Autodesk Inventor part; units mm, degrees
ref_plane "YZ Plane" through (0, 0, 0) normal (1, 0, 0) x (0, 1, 0)
ref_plane "XZ Plane" through (0, 0, 0) normal (0, 1, 0) x (-1, 0, 0)
ref_plane "XY Plane" through (0, 0, 0) normal (0, 0, 1) x (1, 0, 0)
sketch "Sketch1" plane through (0, 0, 0) normal (0, 0, 1) x (1, 0, 0)
  circle A0 centre (0, 0) radius 5
  dimension "d0" = 10
extrude "Extrusion1" add sketch "Sketch1" along normal blind 1
sketch "Sketch2" plane through (0, 0, 1) normal (0, 0, 1) x (1, 0, 0)
  circle A0 centre (0, 0) radius 1.5
  circle A1 centre (0, 0) radius 2
  dimension "d3" = 3
  dimension "d4" = 4
extrude "Extrusion2" cut sketch "Sketch2" against normal blind 1.5 contours A0
extrude "Extrusion3" add sketch "Sketch2" along normal blind 2
mirror "Mirror2" about plane through (0, 0, 0) normal (0, 0, -1)
properties part number "einzel_element"
Source: CAD feature listing. Evaluate the final solid. Frame: model axes, mm. A direction names the side the tool comes from. Round coordinates to 2 decimals unless told otherwise and drop trailing zeros. Loops run counter-clockwise (first coordinate to the right, second up) from the corner with the lowest first, then second, coordinate; pieces in that order, holes last. Notation, with made-up numbers: (52.5, -18.75) - (104.5, -18.75) arc R28 ccw to (104.5, 8.25) - close; hole circle Ø7 at (35.25, 37.25). An arc over 180 degrees is marked (long way). Write item = value, one per line. Start each with the question number.
(1) Set-up query: faces 4 (the face through (0, 2, 2)), 5 (the face through (-1.08, -4.88, 0.01)). Return all of +Z, -Z, +X, -X, +Y, -Y with unobstructed straight access to the full face (end or side cutting, diameter ignored); none if empty.
(2) Section query C-C, the plane z = 1.85. Output: boundary loops of the cut face in (x, y), plus the area to 3 significant figures.
(3) Section query D-D, the plane y = -3. Output: boundary loops of the cut face in (x, z).
(4) Section query A-A, the plane y = 0. Output: boundary loops of the cut face in (x, z).
(5) Pull-direction query (Y, two-part tool) for faces 1 (the face through (-2.2, 0.1, -1)), 2 (the face through (-1.5, 0.07, 0.04)), 3 (the face through (0, -2, -2)); classes: +Y half, -Y half, draft (parallel to the pull), parting line (faces both ways), or undercut.
(6) Ray query, line 1 along Y through (x, z) = (0, 0.5); line 2 along Y through (x, z) = (0, 1.15); line 3 along X through (y, z) = (-1, -1.2). Return the intervals inside material, ascending. Write a range as from..to.
(7) Pin query (flat end, axial travel): pin 1 (2 mm diameter, centred on y = -1.5, z = 1.5, fed in from +X); pin 2 (1.5 mm diameter, centred on x = 2, z = -0.5, fed in from -Y); pin 3 (6 mm diameter, centred on x = 4, y = 1.5, fed in from +Z); pin 4 (2 mm diameter, centred on y = 3.5, z = 1.5, fed in from -X). Return the tip coordinate at first contact, or that it passes through.
Conclusion:
q1.face_4 = +Z
q1.face_5 = +Z, -Z
q2.outline = circle Ø4 at (0, 0); hole circle Ø3 at (0, 0)
q2.area = 5.50 mm2
q3.outline = (-4, -1) - (4, -1) - (4, 1) - (-4, 1) - close
q4.outline = (-5, -1) - (-2, -1) - (-2, -3) - (-1.5, -3) - (-1.5, 3) - (-2, 3) - (-2, 1) - (-5, 1) - close; (1.5, -3) - (2, -3) - (2, -1) - (5, -1) - (5, 1) - (2, 1) - (2, 3) - (1.5, 3) - close
q5.face_1 = draft
q5.face_2 = undercut
q5.face_3 = parting line
q6.line_1 = -5..-1.5, 1.5..5
q6.line_2 = -2..-1.5, 1.5..2
q6.line_3 = -1.73..-1.12, 1.12..1.73
q7.pin_1 = 4.96
q7.pin_2 = -4.84
q7.pin_3 = 3
q7.pin_4 = -4.25
